Design review of the part built by this model. Coordinates are the model's own, in mm. Give positions to 0.01 mm unless a question says otherwise; leave off trailing zeros. Loops run counter-clockwise (first coordinate to the right, second up) from the corner with the lowest first, then second, coordinate; pieces in that order, holes last. Notation, with made-up numbers: M -10.75,-34.75 L 48.25,-34.75 A11 ccw 48.25,-22.75 Z; hole C 69,49 d6. An arc over 180 degrees is marked long. Answer as CSV lines item,"result".
```python
from build123d import *

# Parameters (mm, degrees)
F0_W     = 609.6
F0_H     = 406.4
F1_DEPTH = 4.7625
F3_DEPTH = 25.4
F5_D     = 5.8
F7_DEPTH = 25.4
F9_D     = 4.8
F10_R    = 12.7


with BuildPart() as f1:
    # F0 (on Top) → F1 (new body)
    with BuildSketch(Plane.XY):
        Rectangle(F0_W, F0_H)
    extrude(amount=F1_DEPTH)

    # F2 (on face) → F3 (cut)
    with BuildSketch(Plane.XY.offset(4.7625)):
        Polygon((-152.4, -203.2), (-304.8, -177.8), (-304.8, -203.2), align=None)
        Polygon((152.4, -203.2), (304.8, -203.2), (304.8, -177.8), align=None)
    extrude(amount=-F3_DEPTH, mode=Mode.SUBTRACT)

    # F5 (through all)
    with Locations(Plane.XY.offset(4.7625)):
        with Locations((-206.375, 187.325), (-176.2125, 187.325), (176.2125, 187.325), (206.375, 187.325)):
            Hole(F5_D / 2)

    # F6 (on face) → F7 (cut)
    with BuildSketch(Plane.XY.offset(4.7625)):
        with BuildLine():
            Line((304.8, -127), (304.8, -120.65))
            ThreePointArc((304.8, -120.65), (301.625, -123.825), (304.8, -127))
        make_face()
        with BuildLine():
            Line((304.8, -142.875), (304.8, -136.525))
            ThreePointArc((304.8, -136.525), (301.625, -139.7), (304.8, -142.875))
        make_face()
    extrude(amount=-F7_DEPTH, mode=Mode.SUBTRACT)

    # F9 (through all)
    with Locations(Plane.XY.offset(4.7625)):
        with Locations((287.3375, -139.7)):
            Hole(F9_D / 2)

    # F10
    f10_edges = [f1.edges().sort_by_distance(p)[0] for p in [
        (304.8, -177.8, 2.38125),
        (-304.8, -177.8, 2.38125),
        (304.8, 203.2, 2.38125),
        (-304.8, 203.2, 2.38125),
    ]]
    fillet(f10_edges, radius=F10_R)


solid = f1.part
```
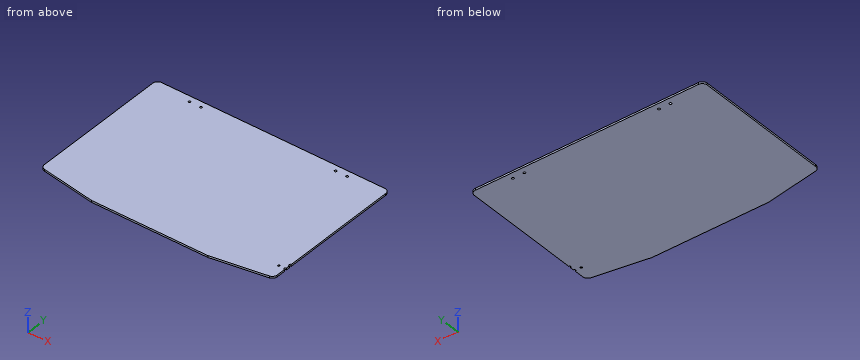
1. We need section C-C, the plane x = 268. Write out the cut boundary in (y, z).
Answer block:
outline,"M -183.93,0 L 203.2,0 L 203.2,4.76 L -183.93,4.76 Z"
2. For P1, Ø5, axis at x = 176.21, y = 187.32, coming from the +Z side, flat-tipped, find the tip position at first contact; note if it passes through.
Answer block:
P1,"through"
3. We need section A-A, the plane z = 2.35. Count the separate pieces of the cut face and the enclosed holes in it, plus the area to 3 significant figures.
Answer block:
separate pieces,"1"
enclosed holes,"5"
area,"244,000 mm²"
4. We need section B-B, the plane x = 192. Write out the cut boundary in (y, z).
Answer block:
outline,"M -196.6,0 L 203.2,0 L 203.2,4.76 L -196.6,4.76 Z"
5. To check wall thickness, follow L1, parallel to X at y = -139.7, z = 3 (1 decimal); L2, parallel to Y at x = -229, z = 1.45; L3, parallel to Y at x = -173, z = 3.9. State the ranges of each line that lie inside material, in increasing order. Write a range as [from, to].
Answer block:
L1,"[-304.8, 284.9], [289.7, 301.6]"
L2,"[-190.43, 203.2]"
L3,"[-199.77, 203.2]"
